```python
from build123d import *

# Parameters (mm, degrees)
SKETCH003_R           = 2.3
SKETCH003_W           = 2
SKETCH003_H           = 5
EXTRUDE003_DEPTH      = 5
EXTRUDE003_DEPTH_BACK = 3
ARRAY001_COUNT        = 4
SKETCH002_R           = 45
SKETCH002_R_2         = 13
EXTRUDE002_DEPTH      = 1


with BuildPart() as array001:
    # Sketch003 → Extrude003 (new body, two sides)
    with BuildSketch(Plane.XY) as extrude003_sk:
        with Locations((0, 38.25)):
            Circle(SKETCH003_R)
        with Locations((0, 10.5)):
            Rectangle(SKETCH003_W, SKETCH003_H)
    extrude(amount=EXTRUDE003_DEPTH)
    extrude(extrude003_sk.sketch, amount=-EXTRUDE003_DEPTH_BACK)

    # Array001: Array001 ×4 about axis
    array001_axis = Axis((0, 0, 0), (0, 0, 1))


with BuildPart() as array001_1:
    add(array001.part)
    for i in range(1, ARRAY001_COUNT):
        add(array001.part.rotate(array001_axis, i * 360 / ARRAY001_COUNT))


with BuildPart() as cut:
    # Sketch002 → Extrude002 (new body, symmetric)
    with BuildSketch(Plane.XY):
        Circle(SKETCH002_R)
        Circle(SKETCH002_R_2, mode=Mode.SUBTRACT)
    extrude(amount=EXTRUDE002_DEPTH, both=True)

    # Cut: cut Array001
    add(array001_1.part, mode=Mode.SUBTRACT)


solid = cut.part
```
Model file for the job. Use its own axes, mm. A direction names the side the tool comes from. Give positions to 0.01 mm unless a question says otherwise; leave off trailing zeros. Order: outer loops, then holes, each group sorted by start corner. A loop starts at its lowest first (then second) coordinate and runs counter-clockwise, first axis right, second up.
1) 3-axis set-ups, long thin cutter, end or side, ignore diameter. For faces 1 (the flat face through (9.4, -9.4, 1)), 2 (the cylindrical face through (9.101, -9.283, -0.014)): which of +Z, -Z, +X, -X, +Y, -Y reach the whole face in a straight line?
2) Saw through at C-C, the plane z = 0.4. Count the separate pieces of the cut face and the enclosed holes in it, then the cut area to 3 significant figures.
3) Saw through at D-D, the plane y = -22.5. Write the cut outline in (x, z), then the cut area to 3 significant figures.
4) Mould opens along X. For faces 3 (the cylindrical face through (20.765, -39.923, 0.014)), 4 (the flat face through (13, 0, 0)), 5 (the flat face through (9.4, -9.4, -1)) say: +X half, -X half, draft (parallel to the pull), parting line (faces both ways), or undercut.
5) Wall check: probe 1 along Y at (x, z) = (0, -0.2); probe 2 along Y at (x, z) = (-3, -0.45); probe 3 along Y at (x, z) = (-38.25, -0.6). Give the ranges that are in metal, low to high.
6) Saw through at B-B, the plane y = -8.5. Write the cut outline in (x, z).
7) Pin check, flat tips, straight feed: pin 1 (1 mm diameter, centred on x = 0, z = 0, fed in from -Y); pin 2 (0.6 mm diameter, centred on x = 0.5, z = 0, fed in from +Y); pin 3 (1 mm diameter, centred on x = -33, z = 0.5, fed in from +Y). Stop position of each tip, or through.
8) Saw through at A-A, the plane x = -9.5. Write the cut outline in (y, z).
Computed:
1. face 1: +Z, +X, -X, +Y, -Y
1. face 2: +Z, -Z
2. separate pieces: 1
2. enclosed holes: 5
2. area: 5,760 mm2
3. outline: (-38.97, -1) - (38.97, -1) - (38.97, 1) - (-38.97, 1) - close
3. area: 156 mm2
4. face 3: parting line
4. face 4: undercut
4. face 5: draft
5. probe 1: y = -45 to -40.55, -35.95 to -13, 13 to 35.95, 40.55 to 45
5. probe 2: y = -44.9 to -12.65, 12.65 to 44.9
5. probe 3: y = -23.71 to -2.3, 2.3 to 23.71
6. outline: (-44.19, -1) - (-9.84, -1) - (-9.84, 1) - (-44.19, 1) - close; (9.84, -1) - (44.19, -1) - (44.19, 1) - (9.84, 1) - close
7. pin 1: stops at y = -45
7. pin 2: stops at y = 45
7. pin 3: stops at y = 31.12
8. outline: (-43.99, -1) - (-8.87, -1) - (-8.87, 1) - (-43.99, 1) - close; (8.87, -1) - (43.99, -1) - (43.99, 1) - (8.87, 1) - close
